Work out the finished part from the listing and answer in its coordinate system (mm). Coordinates: 2 decimals unless noted, no trailing zeros. Write each loop counter-clockwise with the first axis right and the second up, starting at its lowest first coordinate (ties: lowest second). Pieces come first, ordered by that corner, then holes. Notation, with made-up numbers: (70, 61.5) - (118, 61.5) arc R24 ccw to (118, 81.5) - close; hole circle Ø2 at (-21.75, 79). An arc over 180 degrees is marked (long way). Use CSV: the item, a comma, the result in double quotes. Start each with the question number.
from build123d import *

# Parameters (mm, degrees)
SKETCH1_R           = 2.5
BOSS_EXTRUDE1_DEPTH = 2.5


with BuildPart() as part:
    # Sketch1 → Boss-Extrude1 (new body)
    with BuildSketch(Plane(origin=(0, 0, -1.25), x_dir=(-1, 0, 0), z_dir=(0, 0, -1))):
        Polygon((-2.908088852, -12.7), (88.646, -12.7), (94.996, -6.35), (94.996, 6.35), (85.443949258, 41.998738686), (79.093949258, 52.997261314), (70.419687944, 55.321522628), (-8.868478822, 9.544478202), align=None)
        with Locations((25.4, 0)):
            Circle(SKETCH1_R, mode=Mode.SUBTRACT)
        with Locations((38.1, 0)):
            Circle(SKETCH1_R, mode=Mode.SUBTRACT)
        with Locations((50.8, 0)):
            Circle(SKETCH1_R, mode=Mode.SUBTRACT)
        with Locations((63.5, 0)):
            Circle(SKETCH1_R, mode=Mode.SUBTRACT)
        Circle(SKETCH1_R, mode=Mode.SUBTRACT)
        with Locations((88.9, 0)):
            Circle(SKETCH1_R, mode=Mode.SUBTRACT)
        with Locations((76.2, 0)):
            Circle(SKETCH1_R, mode=Mode.SUBTRACT)
        with Locations((76.989658396, 44.45)):
            Circle(SKETCH1_R, mode=Mode.SUBTRACT)
        with Locations((65.991135768, 38.1)):
            Circle(SKETCH1_R, mode=Mode.SUBTRACT)
        with Locations((54.99261314, 31.75)):
            Circle(SKETCH1_R, mode=Mode.SUBTRACT)
        with Locations((43.994090512, 25.4)):
            Circle(SKETCH1_R, mode=Mode.SUBTRACT)
        with Locations((32.995567884, 19.05)):
            Circle(SKETCH1_R, mode=Mode.SUBTRACT)
        with Locations((21.997045256, 12.7)):
            Circle(SKETCH1_R, mode=Mode.SUBTRACT)
        with BuildLine():
            Line((10.285185434, -0.647047613), (8.583708062, 5.702952387))
            ThreePointArc((8.583708062, 5.702952387), (10.351475015, 8.764814566), (13.413337194, 6.997047613))
            Line((13.413337194, 6.997047613), (15.114814566, 0.647047613))
            ThreePointArc((15.114814566, 0.647047613), (13.347047613, -2.414814566), (10.285185434, -0.647047613))
        make_face(mode=Mode.SUBTRACT)
    extrude(amount=-BOSS_EXTRUDE1_DEPTH)


solid = part.part
Item 1: A cutting plane is placed at B-B (y = 25.4). Determine the outline of the cut face in (x, z).
Item 2: Straight lines are drawn through the part: probe 1 along Y at (x, z) = (-23.5, 0.55); probe 2 along Y at (x, z) = (-65.5, -0.15); probe 3 along Y at (x, z) = (-68, 0.2). For each, find the intervals that lie inside material, in ascending order. Write a range as [from, to].
Item 3: Determine the mould class of faces 1 (the face through (-94.996, 0, 0)), 2 (the face through (5.93, -1.42, -0.02)), 3 (the face through (-35.305, 18.092, -0.018)) for opening direction X: +X half, -X half, draft (parallel to the pull), parting line (faces both ways), or undercut.
Item 4: A cutting plane is placed at A-A (z = 0.8). Count the separate pieces of the cut face and the enclosed holes in it, then the cut area to 3 significant figures.
Item 5: A cutting plane is placed at D-D (x = -38.1). Determine the outline of the cut face in (y, z).
Item 6: A cutting plane is placed at C-C (x = -76.2). Determine the outline of the cut face in (y, z).
Calculated:
1,outline,"(-89.89, -1.25) - (-46.49, -1.25) - (-46.49, 1.25) - (-89.89, 1.25) - close; (-41.49, -1.25) - (-18.59, -1.25) - (-18.59, 1.25) - (-41.49, 1.25) - close"
2,probe 1,"y = [-12.7, -1.62], [1.62, 10.7], [14.7, 28.23]"
2,probe 2,"y = [-12.7, -1.5], [1.5, 35.65], [40.55, 52.48]"
2,probe 3,"y = [-12.7, 36.61], [39.59, 53.92]"
3,face 1,"-X half"
3,face 2,"+X half"
3,face 3,"undercut"
4,separate pieces,"1"
4,enclosed holes,"14"
4,area,"4,500 mm²"
5,outline,"(-12.7, -1.25) - (-2.5, -1.25) - (-2.5, 1.25) - (-12.7, 1.25) - close; (2.5, -1.25) - (36.66, -1.25) - (36.66, 1.25) - (2.5, 1.25) - close"
6,outline,"(-12.7, -1.25) - (-2.5, -1.25) - (-2.5, 1.25) - (-12.7, 1.25) - close; (2.5, -1.25) - (42.08, -1.25) - (42.08, 1.25) - (2.5, 1.25) - close; (46.82, -1.25) - (53.77, -1.25) - (53.77, 1.25) - (46.82, 1.25) - close"
